Can you work these out from the model? Positions are in its coordinate system, mm. A direction names the side the tool comes from. Round coordinates to 2 decimals unless told otherwise and drop trailing zeros. Order: outer loops, then holes, each group sorted by start corner. A loop starts at its lowest first (then second) coordinate and runs counter-clockwise, first axis right, second up.
Q1. If I drill on line 1 (Y direction, x = -122.75, z = 45); line 2 (Y direction, x = -121.5, z = 13.5); line 3 (X direction, y = 0.75, z = 54), over which ranges is the centre line in solid material (lowest first)?
Q2. If we section it at B-B (x = -121.5): Please give me the cut outline in (y, z).
Q3. If we section it at D-D (z = 32): Please give me the cut outline in (x, y).
Q4. For faces 4 (the face through (-125.874, 2.012, 12.675)), 5 (the face through (-124.745, 0, 51)), 6 (the face through (-123.976, 0.067, 54.108)), which set-ups out of +Z, -Z, +X, -X, +Y, -Y let a thin tool reach every point of the face, with its end or its side?
Q5. If we section it at C-C (z = 25.5): Please give me the cut outline in (x, y).
Q6. Will these pins go through, and if not, where does the flat tip stop? P1, Ø0.8, axis at y = 0, z = 40.5, coming from the -X side; P2, Ø1.2, axis at y = -2, z = 60.5, coming from the -X side; P3, Ø1.6, axis at y = -1.5, z = 5.5, coming from the -X side.
Q7. We'd pull the mould along Z, two halves only. Please class faces 1 (the face through (-120, 0, 63.5)), 2 (the face through (-125.874, 2.012, 32.995)), 3 (the face through (-126, 0, 24.65)): pulls with the +Z half, pulls with the -Z half, needs draft (parallel to the pull), parting line crosses it, or undercut.
Q8. If we section it at A-A (z = 53.5): Please give me the cut outline in (x, y).
from build123d import *

# Parameters (mm, degrees)
BOSS_EXTRUDE1_DEPTH = 63.5
SKETCH2_R           = 1.524
CUT_EXTRUDE1_DEPTH  = 19.05
CUT_EXTRUDE2_START  = -19.05
SKETCH3_R           = 1.524
CUT_EXTRUDE2_DEPTH  = 19.05
SKETCH6_W           = 2.291358881
SKETCH6_H           = 1.5
CUT_EXTRUDE4_DEPTH  = 19.05


with BuildPart() as part:
    # Sketch1 → Boss-Extrude1 (new body)
    with BuildSketch(Plane.XY):
        Polygon((-117.870682238, 0), (-120.162041119, 3.96875), (-124.744758881, 3.96875), (-127.036117762, 0), (-124.744758881, -3.96875), (-120.162041119, -3.96875), align=None)
    extrude(amount=BOSS_EXTRUDE1_DEPTH)

    # Sketch2 → Cut-Extrude1 (cut)
    with BuildSketch(Plane.XY.offset(63.5)):
        with Locations((-122.4534, 0)):
            Circle(SKETCH2_R)
    extrude(amount=-CUT_EXTRUDE1_DEPTH, mode=Mode.SUBTRACT)

    # Sketch3 → Cut-Extrude2 (cut)
    with BuildSketch(Plane(origin=(0, 0, 0), x_dir=(-1, 0, 0), z_dir=(0, 0, -1)).offset(CUT_EXTRUDE2_START)):
        with Locations(Location((122.4534, 0, 0), (0, 0, 180))):
            Circle(SKETCH3_R)
    extrude(amount=CUT_EXTRUDE2_DEPTH, mode=Mode.SUBTRACT)

    # Sketch6 → Cut-Extrude4 (cut)
    with BuildSketch(Plane.XZ.offset(3.96875)):
        with Locations((-125.890438321, 5.08)):
            Rectangle(SKETCH6_W, SKETCH6_H)
        with Locations((-125.890438321, 10.16)):
            Rectangle(SKETCH6_W, SKETCH6_H)
        with Locations((-125.890438321, 15.24)):
            Rectangle(SKETCH6_W, SKETCH6_H)
        with Locations((-125.890438321, 20.32)):
            Rectangle(SKETCH6_W, SKETCH6_H)
        with Locations((-125.890438321, 25.4)):
            Rectangle(SKETCH6_W, SKETCH6_H)
        with Locations((-125.890438321, 30.48)):
            Rectangle(SKETCH6_W, SKETCH6_H)
        with Locations((-125.890438321, 35.56)):
            Rectangle(SKETCH6_W, SKETCH6_H)
        with Locations((-125.890438321, 40.64)):
            Rectangle(SKETCH6_W, SKETCH6_H)
        with Locations((-125.890438321, 45.72)):
            Rectangle(SKETCH6_W, SKETCH6_H)
        with Locations((-125.890438321, 50.8)):
            Rectangle(SKETCH6_W, SKETCH6_H)
        with Locations((-125.890438321, 55.88)):
            Rectangle(SKETCH6_W, SKETCH6_H)
        with Locations((-125.890438321, 60.96)):
            Rectangle(SKETCH6_W, SKETCH6_H)
        with Locations((-125.890438321, 66.04)):
            Rectangle(SKETCH6_W, SKETCH6_H)
        with Locations((-125.890438321, 71.12)):
            Rectangle(SKETCH6_W, SKETCH6_H)
    extrude(amount=-CUT_EXTRUDE4_DEPTH, mode=Mode.SUBTRACT)


solid = part.part
Solution:
1. line 1: y = -3.97 to -1.49, 1.49 to 3.97
1. line 2: y = -3.97 to -1.19, 1.19 to 3.97
1. line 3: x = -126.6 to -123.78, -121.13 to -118.3
2. outline: (-3.97, 0) - (-1.19, 0) - (-1.19, 19.05) - (1.19, 19.05) - (1.19, 0) - (3.97, 0) - (3.97, 63.5) - (1.19, 63.5) - (1.19, 44.45) - (-1.19, 44.45) - (-1.19, 63.5) - (-3.97, 63.5) - close
3. outline: (-127.04, 0) - (-124.74, -3.97) - (-120.16, -3.97) - (-117.87, 0) - (-120.16, 3.97) - (-124.74, 3.97) - close
4. face 4: +Z, -Z, -X, +Y
4. face 5: -X, +Y, -Y
4. face 6: +Z
5. outline: (-124.74, -3.97) - (-120.16, -3.97) - (-117.87, 0) - (-120.16, 3.97) - (-124.74, 3.97) - close
6. P1: stops at x = -124.74
6. P2: stops at x = -126.18
6. P3: stops at x = -126.59
7. face 1: pulls with the +Z half
7. face 2: needs draft
7. face 3: undercut
8. outline: (-127.04, 0) - (-124.74, -3.97) - (-120.16, -3.97) - (-117.87, 0) - (-120.16, 3.97) - (-124.74, 3.97) - close; hole circle Ø3.05 at (-122.45, 0)
